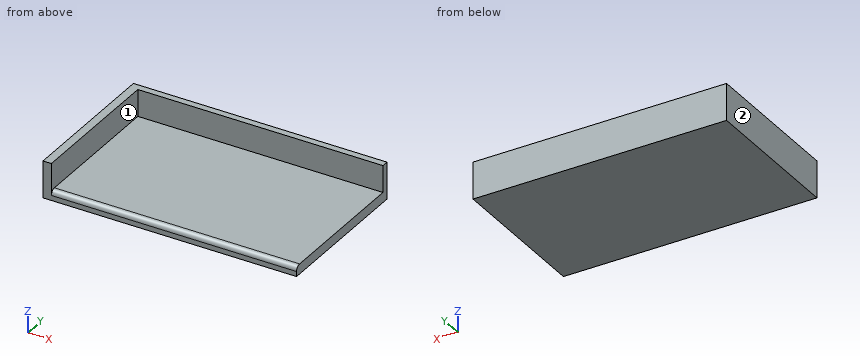
from build123d import *

# Parameters (mm, degrees)
F0_W          = 927.1
F0_H          = 38.1
F1_DEPTH      = 542.925
F3_W          = 31.75
F3_H          = 568.325
F4_DEPTH      = 120.65
F4_DEPTH_BACK = 19.05
F5_W          = 927.1
F5_H          = 25.4
F6_DEPTH      = 120.65
F6_DEPTH_BACK = 19.05
F7_R          = 19.05


with BuildPart() as f1:
    # F0 (on Front) → F1 (new body)
    with BuildSketch(Plane.XZ):
        Rectangle(F0_W, F0_H)
    extrude(amount=F1_DEPTH)

    # F3 (on Top) → F4 (join, two sides)
    with BuildSketch(Plane.XY) as f4_sk:
        with Locations((-479.425, -258.7625)):
            Rectangle(F3_W, F3_H)
    extrude(amount=F4_DEPTH)
    extrude(f4_sk.sketch, amount=-F4_DEPTH_BACK)

    # F5 (on Top) → F6 (join, two sides)
    with BuildSketch(Plane.XY) as f6_sk:
        with Locations((0, 12.7)):
            Rectangle(F5_W, F5_H)
    extrude(amount=F6_DEPTH)
    extrude(f6_sk.sketch, amount=-F6_DEPTH_BACK)

    # F7
    f7_edges = [f1.edges().sort_by_distance(p)[0] for p in [
        (0, -542.925, 19.05),
    ]]
    fillet(f7_edges, radius=F7_R)


solid = f1.part
Work out the finished part from the listing and answer in its coordinate system (mm). Face numbers are marked on the shaded views. A direction names the side the tool comes from. Round coordinates to 2 decimals unless told otherwise and drop trailing zeros. Loops run counter-clockwise (first coordinate to the right, second up) from the corner with the lowest first, then second, coordinate; pieces in that order, holes last. Notation, with made-up numbers: M 62,72.5 L 74,72.5 A20 ccw 74,86.5 Z; hole C -5.75,-37.75 d2. An arc over 180 degrees is marked long. One line per question, with ' | ' between items. Start each with the question number.
(1) Flat-ended cylindrical pins translate along their axes: pin 1 Ø2 at (x, z) = (-329.5, 21.5) entering from -Y; pin 2 Ø10 at (x, z) = (-277, 8) entering from -Y; pin 3 Ø3 at (y, z) = (-347.5, 33) entering from +X. Find the tip coordinate at first contact, or state that the pin passes through.
(2) A cutting plane is placed at C-C on z = 106.5. Write down the section's boundary in (x, y) (3 decimals).
(3) Find the intervals of material crossed by line 1 (X direction, y = -7.5, z = 26); line 2 (Z direction, x = 289, y = -131.5), in increasing order.
(4) A tool of negligible diameter and unlimited length cuts with its end or side. For the marked faces 1 and 2, from which of +Z, -Z, +X, -X, +Y, -Y can it reach the whole face along a straight path? Write none if from no direction.
(5) A cutting plane is placed at A-A on y = -286. Write down the section's boundary in (x, z).
(6) A cutting plane is placed at B-B on x = 163.5. Write down the section's boundary in (y, z) (3 decimals).
Geometry check:
1) pin 1: stops at y = 0 | pin 2: stops at y = -542.69 | pin 3: stops at x = -463.55
2) outline: M -495.3,-542.925 L -463.55,-542.925 L -463.55,0 L 463.55,0 L 463.55,25.4 L -495.3,25.4 Z
3) line 1: x = -495.3 to -463.55 | line 2: z = -19.05 to 19.05
4) face 1: +Z, +X, -Y | face 2: +Z, -Z, -X, +Y, -Y
5) outline: M -495.3,-19.05 L 463.55,-19.05 L 463.55,19.05 L -463.55,19.05 L -463.55,120.65 L -495.3,120.65 Z
6) outline: M -542.925,-19.05 L 25.4,-19.05 L 25.4,120.65 L 0,120.65 L 0,19.05 L -523.875,19.05 A19.05 ccw -542.925,0 Z
